For this review, take the finished solid that the model builds, in its own axes (mm). A direction names the side the tool comes from. Give positions to 0.01 mm unless a question says otherwise; leave off trailing zeros. Loops run counter-clockwise (first coordinate to the right, second up) from the corner with the lowest first, then second, coordinate; pieces in that order, holes last. Notation, with made-up numbers: (-13.75, -20.5) - (14.25, -20.5) arc R17 ccw to (14.25, -14.5) - close; hole circle Ø4 at (40, 73). An arc over 180 degrees is marked (long way). Use CSV: the item, a comma, the result in double quotes. Start each with the question number.
1. Take a section at D-D on x = 8.5. Give the boundary of the cut face in (y, z), plus the area to 3 significant figures.
2. For faces 4 (the flat face through (13.5, -4.4, 5.5)), 5 (the flat face through (-7, -3.2, 7)), list the 3-axis set-ups (+Z, -Z, +X, -X, +Y, -Y) from which the entire face can be reached by the end or side of a thin tool; tool diameter is ignored.
3. Take a section at C-C on z = 0.5. Give the boundary of the cut face in (x, y).
4. Take a section at A-A on y = 0. Give the boundary of the cut face in (x, z).
5. Wall thickness on line 1 (Y direction, x = 0, z = 6.75); line 2 (Y direction, x = 0, z = 2.75); line 3 (X direction, y = -6, z = 3): over which ranges is each line inside the solid? List them lowest first.
6. Mouldability with a two-part tool opening along X and no side actions: class faces 1 (the cylindrical face through (7.493, 0.33, 3.451)), 2 (the cylindrical face through (-12.1, -9.28, 6.24)), 3 (the flat face through (6, -6, 0)) as pulls with the +X half, pulls with the -X half, needs draft (parallel to the pull), parting line crosses it, or undercut.
7. For pin 1 (1.5 mm diameter, centred on y = 5, z = 5, fed in from +X); pin 2 (1 mm diameter, centred on x = -8.5, z = 4.5, fed in from -Y), all flat-tipped, find the tip position at first contact; note any pin that passes through.
```python
from build123d import *

# Parameters (mm, degrees)
SKETCH_1_R          = 14
EXTRUDE_1_DEPTH     = 5.5
SKETCH_2_R          = 15.25
EXTRUDE_2_DEPTH     = 1.5
CUT_EXTRUDE_1_REACH = 9
SKETCH_3_R          = 7.5


with BuildPart() as part:
    # 草图1 → 凸台-拉伸1 (new body)
    with BuildSketch(Plane.XY):
        Circle(SKETCH_1_R)
    extrude(amount=EXTRUDE_1_DEPTH)

    # 草图2 → 凸台-拉伸2 (add)
    with BuildSketch(Plane.XY.offset(5.5)):
        Circle(SKETCH_2_R)
    extrude(amount=EXTRUDE_2_DEPTH)

    # 草图3 → 切除-拉伸1 (cut, up to next)
    with BuildSketch(Plane(origin=(0, 0, 0), x_dir=(-1, 0, 0), z_dir=(0, 0, -1)), mode=Mode.PRIVATE) as cut_extrude_1_sk1:
        Circle(SKETCH_3_R)
    cut_extrude_1_tool1 = extrude(cut_extrude_1_sk1.sketch, amount=-CUT_EXTRUDE_1_REACH, mode=Mode.PRIVATE) & part.part
    add(cut_extrude_1_tool1.solids().sort_by_distance((0, 0, 0))[0], mode=Mode.SUBTRACT)


solid = part.part
```
Check result:
1,outline,"(-12.66, 5.5) - (-11.12, 5.5) - (-11.12, 0) - (11.12, 0) - (11.12, 5.5) - (12.66, 5.5) - (12.66, 7) - (-12.66, 7) - close"
1,area,"160 mm²"
2,face 4,"-Z"
2,face 5,"+Z, +X, -X, +Y, -Y"
3,outline,"circle Ø28 at (0, 0); hole circle Ø15 at (0, 0)"
4,outline,"(-15.25, 5.5) - (-14, 5.5) - (-14, 0) - (-7.5, 0) - (-7.5, 7) - (-15.25, 7) - close; (7.5, 0) - (14, 0) - (14, 5.5) - (15.25, 5.5) - (15.25, 7) - (7.5, 7) - close"
5,line 1,"y = -15.25 to -7.5, 7.5 to 15.25"
5,line 2,"y = -14 to -7.5, 7.5 to 14"
5,line 3,"x = -12.65 to -4.5, 4.5 to 12.65"
6,face 1,"undercut"
6,face 2,"parting line crosses it"
6,face 3,"needs draft"
7,pin 1,"stops at x = 14.59"
7,pin 2,"stops at y = -11.49"
